from build123d import *
from build123d.topology import SkipClean

# Parameters (mm, degrees)
SKETCH1_R           = 15
SKETCH1_R_2         = 10
SKETCH1_R_3         = 6
BOSS_EXTRUDE1_DEPTH = 5
BOSS_EXTRUDE2_START = 2.5
SKETCH2_R           = 15
SKETCH2_R_2         = 10
BOSS_EXTRUDE2_DEPTH = 2.5
BOSS_EXTRUDE4_START = 3
BOSS_EXTRUDE4_DEPTH = 3


with BuildPart() as part:
    # Sketch1 → Boss-Extrude1 (new body)
    # profile 1 of 2: a face of its own
    with BuildSketch(Plane.XY):
        Circle(SKETCH1_R)
        Circle(SKETCH1_R_2, mode=Mode.SUBTRACT)
    # profile 2 of 2: a face of its own
    with BuildSketch(Plane.XY):
        Circle(SKETCH1_R_2)
        Circle(SKETCH1_R_3, mode=Mode.SUBTRACT)
    extrude(amount=-BOSS_EXTRUDE1_DEPTH)

    # Sketch2 → Boss-Extrude2 (add)
    with BuildSketch(Plane.XY.offset(BOSS_EXTRUDE2_START)):
        Circle(SKETCH2_R)
        Circle(SKETCH2_R_2, mode=Mode.SUBTRACT)
    extrude(amount=-BOSS_EXTRUDE2_DEPTH)

    # Sketch3 → Boss-Extrude4 (add)
    with SkipClean():  # the faces are left unmerged after this step: merging them gives an invalid solid
        with BuildSketch(Plane.XY.offset(2.5).offset(BOSS_EXTRUDE4_START)):
            with BuildLine():
                ThreePointArc((-2.290603582, -14.824072829), (0, -15), (2.290603582, -14.824072829))
                ThreePointArc((2.290603582, -14.824072829), (3.086155614, -13.560105094), (3.235238064, -12.074072829))
                ThreePointArc((3.235238064, -12.074072829), (2.788392741, -10.80499404), (1.867509855, -9.824072829))
                ThreePointArc((1.867509855, -9.824072829), (0, -10), (-1.867509855, -9.824072829))
                ThreePointArc((-1.867509855, -9.824072829), (-2.788392741, -10.80499404), (-3.235238064, -12.074072829))
                ThreePointArc((-3.235238064, -12.074072829), (-3.086155614, -13.560105094), (-2.290603582, -14.824072829))
            make_face()
            with BuildLine():
                ThreePointArc((-14.806366496, -2.402396967), (-14.265847744, -4.635254916), (-13.390695627, -6.759383893))
                ThreePointArc((-13.390695627, -6.759383893), (-11.942751779, -7.125411327), (-10.483382099, -6.807987938))
                ThreePointArc((-10.483382099, -6.807987938), (-9.414499246, -5.990845869), (-8.766156198, -4.811912875))
                ThreePointArc((-8.766156198, -4.811912875), (-9.510565163, -3.090169944), (-9.920340763, -1.259698041))
                ThreePointArc((-9.920340763, -1.259698041), (-11.137820734, -0.687007696), (-12.482869184, -0.654199453))
                ThreePointArc((-12.482869184, -0.654199453), (-13.850100843, -1.255194512), (-14.806366496, -2.402396967))
            make_face()
            with BuildLine():
                ThreePointArc((-6.860234162, 13.339309849), (-8.816778784, 12.135254916), (-10.566508613, 10.64654384))
                ThreePointArc((-10.566508613, 10.64654384), (-10.467182133, 9.15635871), (-9.714324518, 7.866504888))
                ThreePointArc((-9.714324518, 7.866504888), (-8.606873263, 7.102447672), (-7.285292336, 6.850147121))
                ThreePointArc((-7.285292336, 6.850147121), (-5.877852523, 8.090169944), (-4.263597916, 9.045536624))
                ThreePointArc((-4.263597916, 9.045536624), (-4.095159033, 10.380399934), (-4.479599369, 11.669755331))
                ThreePointArc((-4.479599369, 11.669755331), (-5.473677455, 12.784352223), (-6.860234162, 13.339309849))
            make_face()
            with BuildLine():
                ThreePointArc((10.566508613, 10.64654384), (8.816778784, 12.135254916), (6.860234162, 13.339309849))
                ThreePointArc((6.860234162, 13.339309849), (5.473677455, 12.784352223), (4.479599369, 11.669755331))
                ThreePointArc((4.479599369, 11.669755331), (4.095159033, 10.380399934), (4.263597916, 9.045536624))
                ThreePointArc((4.263597916, 9.045536624), (5.877852523, 8.090169944), (7.285292336, 6.850147121))
                ThreePointArc((7.285292336, 6.850147121), (8.606873263, 7.102447672), (9.714324518, 7.866504888))
                ThreePointArc((9.714324518, 7.866504888), (10.467182133, 9.15635871), (10.566508613, 10.64654384))
            make_face()
            with BuildLine():
                ThreePointArc((13.390695627, -6.759383893), (14.265847744, -4.635254916), (14.806366496, -2.402396967))
                ThreePointArc((14.806366496, -2.402396967), (13.850100843, -1.255194512), (12.482869184, -0.654199453))
                ThreePointArc((12.482869184, -0.654199453), (11.137820734, -0.687007696), (9.920340763, -1.259698041))
                ThreePointArc((9.920340763, -1.259698041), (9.510565163, -3.090169944), (8.766156198, -4.811912875))
                ThreePointArc((8.766156198, -4.811912875), (9.414499246, -5.990845869), (10.483382099, -6.807987938))
                ThreePointArc((10.483382099, -6.807987938), (11.942751779, -7.125411327), (13.390695627, -6.759383893))
            make_face()
        extrude(amount=-BOSS_EXTRUDE4_DEPTH)


solid = part.part
Work out the finished part from the listing and answer in its coordinate system (mm). A direction names the side the tool comes from. Coordinates: 2 decimals unless noted, no trailing zeros. Write each loop counter-clockwise with the first axis right and the second up, starting at its lowest first coordinate (ties: lowest second). Pieces come first, ordered by that corner, then holes.
1. The part is cut by section C-C, the plane x = 0. Write down the section's boundary in (y, z), and give its area (3 significant figures).
Results list:
outline: (-15, -5) - (-6, -5) - (-6, 0) - (-10, 0) - (-10, 5.5) - (-15, 5.5) - close; (6, -5) - (15, -5) - (15, 2.5) - (10, 2.5) - (10, 0) - (6, 0) - close
area: 130 mm2
2. For a pull along X with two mould halves and no side action, classify faces 3 (the flat face through (-0.2, -6.5, -5)), 4 (the flat face through (0, 13, 2.5)) as +X half, -X half, draft (parallel to the pull), parting line (faces both ways), or undercut.
Results list:
face 3: draft
face 4: undercut
3. The part is cut by section D-D, the plane z = -0.75. Write down the section's boundary in (x, y), and give its area (3 significant figures).
Results list:
outline: circle Ø30 at (0, 0); hole circle Ø12 at (0, 0)
area: 594 mm2
4. For faces 1 (the flat face through (-12, -4, 5.5)), 2 (the flat face through (0, -7, 0)), determine the directions among +Z, -Z, +X, -X, +Y, -Y from which every point of the face is accessible in a straight line to the end or side of a thin tool.
Results list:
face 1: +Z, +X, -X, +Y, -Y
face 2: +Z
5. Flat-ended cylindrical pins translate along their axes: pin 1 (3 mm diameter, centred on x = 6, z = 3, fed in from -Y); pin 2 (2.5 mm diameter, centred on x = -10, y = 2, fed in from +Z); pin 3 (6 mm diameter, centred on x = 2.5, y = 0, fed in from +Z); pin 4 (5 mm diameter, centred on x = 10.5, z = -2, fed in from +Y). Find the tip coordinate at first contact, or state that the pin passes through.
Results list:
pin 1: stops at y = -14.28
pin 2: stops at z = 2.5
pin 3: passes through
pin 4: stops at y = 12.69
6. The part is cut by section B-B, the plane y = 0. Write down the section's boundary in (x, z), and give its area (3 significant figures).
Results list:
outline: (-15, -5) - (-6, -5) - (-6, 0) - (-10, 0) - (-10, 2.5) - (-15, 2.5) - close; (6, -5) - (15, -5) - (15, 2.5) - (10, 2.5) - (10, 0) - (6, 0) - close
area: 115 mm2
7. Consider line 1 along Y through (x, z) = (0, -2.7); line 2 along Y through (x, z) = (0, 1.7); line 3 along Z through (x, y) = (-10, 1). Determine where each line is inside the solid, lowest interval first.
Results list:
line 1: y = -15 to -6, 6 to 15
line 2: y = -15 to -10, 10 to 15
line 3: z = -5 to 2.5
8. The part is cut by section A-A, the plane z = 3. Write down the section's boundary in (x, y), and give its area (3 significant figures).
Results list:
outline: (-14.81, -2.4) arc R15 ccw to (-13.39, -6.76) arc R3.26 ccw to (-8.77, -4.81) arc R10 cw to (-9.92, -1.26) arc R3.26 ccw to start; (-10.57, 10.65) arc R3.26 ccw to (-7.29, 6.85) arc R10 cw to (-4.26, 9.05) arc R3.26 ccw to (-6.86, 13.34) arc R15 ccw to start; (-2.29, -14.82) arc R15 ccw to (2.29, -14.82) arc R3.26 ccw to (1.87, -9.82) arc R10 cw to (-1.87, -9.82) arc R3.26 ccw to start; (4.26, 9.05) arc R10 cw to (7.29, 6.85) arc R3.26 ccw to (10.57, 10.65) arc R15 ccw to (6.86, 13.34) arc R3.26 ccw to start; (8.77, -4.81) arc R3.26 ccw to (13.39, -6.76) arc R15 ccw to (14.81, -2.4) arc R3.26 ccw to (9.92, -1.26) arc R10 cw to start
area: 145 mm2
